Could you check a few things on this model? Use its own coordinates, in mm. A direction names the side the tool comes from. Give positions to 0.01 mm unless a question says otherwise; leave off trailing zeros. Order: outer loops, then holes, each group sorted by start corner. A loop starts at its lowest first (then second) coordinate and runs counter-clockwise, first axis right, second up. Notation, with made-up numbers: M 74.5,-16 L 93.5,-16 A19 ccw 93.5,-7 Z; hole C 11,-18 d4. An arc over 180 degrees is marked long. Answer in a Markdown table with one row per item. Add a question column.
Autodesk Inventor part; units mm, degrees
ref_plane "YZ Plane" through (0, 0, 0) normal (1, 0, 0) x (0, 1, 0)
ref_plane "XZ Plane" through (0, 0, 0) normal (0, 1, 0) x (-1, 0, 0)
ref_plane "XY Plane" through (0, 0, 0) normal (0, 0, 1) x (1, 0, 0)
sketch "Boceto1" plane through (0, 0, 0) normal (0, 0, 1) x (1, 0, 0)
  line L0 (0, 0) -> (42, 0)
  line L1 (42, 0) -> (42, 42)
  line L2 (42, 42) -> (35, 42)
  line L3 (35, 42) -> (35, 7)
  line L4 (35, 7) -> (0, 7)
  line L5 (0, 7) -> (0, 0)
  dimension "d0" = 7
  dimension "d1" = 7
  dimension "d2" = 42
  dimension "d3" = 42
extrude "Extrusión1" add sketch "Boceto1" along normal blind 41.5
sketch "Boceto2" plane through (0, 0, 41.5) normal (0, 0, 1) x (1, 0, 0)
  line L0 (35, 7) -> (0, 7)
  line L1 (35, 7) -> (35, 38)
  line L2 (35, 42) -> (35, 7)
  line L3 (35, 38) -> (4, 7)
  line L4 (4, 7) -> (35, 7)
  line L5 (42, 42) -> (35, 42)
  point P0 (0, 0)
  point P1 (4, 7)
  dimension "d6" = 4
  dimension "d7" = 4
extrude "Extrusión2" add sketch "Boceto2" against normal blind 4
sketch "Boceto3" plane through (0, 0, 0) normal (0, 0, -1) x (-1, 0, 0)
  line L0 (-4, 7) -> (-35, 38)
  line L1 (-35, 42) -> (-35, 7)
  line L2 (-35, 7) -> (0, 7)
  point P0 (0, 0)
extrude "Extrusión3" add sketch "Boceto3" against normal blind 4
sketch "Boceto4" plane through (35, 42, 0) normal (-1, 0, 0) x (0, 0, 1)
  line L0 (20.75, -11.35) -> (20.75, -22.65) construction
  line L1 (16.4, -11.35) -> (16.4, -22.65)
  line L2 (25.1, -22.65) -> (25.1, -11.35)
  arc A0 (25.1, -11.35) -> (16.4, -11.35) centre (20.75, -11.35) ccw
  arc A1 (16.4, -22.65) -> (25.1, -22.65) centre (20.75, -22.65) ccw
  line L3 (0, 0) -> (41.5, 0)
  point P0 (0, -42)
  point P1 (20.75, -17)
  point P2 (20.75, 0)
  point P3 (20.75, -27)
  point P4 (20.75, -7)
  dimension "d12" = 8.7
  dimension "d13" = 20
  dimension "d14" = 7
extrude "Extrusión4" cut sketch "Boceto4" against normal through all
sketch "Boceto5" plane through (0, 7, 41.5) normal (0, 1, 0) x (1, 0, 0)
  line L0 (22.65, 20.75) -> (11.35, 20.75) construction
  line L1 (22.65, 25.1) -> (11.35, 25.1)
  line L2 (11.35, 16.4) -> (22.65, 16.4)
  arc A0 (22.65, 16.4) -> (22.65, 25.1) centre (22.65, 20.75) ccw
  arc A1 (11.35, 25.1) -> (11.35, 16.4) centre (11.35, 20.75) ccw
  line L3 (0, 41.5) -> (0, 0)
  point P0 (17, 20.75)
  point P1 (0, 20.75)
  point P2 (27, 20.75)
  point P3 (7, 20.75)
  dimension "d17" = 20
  dimension "d18" = 7
  dimension "d19" = 8.7
extrude "Extrusión5" cut sketch "Boceto5" against normal blind 10
properties part number "escuadra pequeña"
1. Suppose I cut it at D-D on x = 8. List the corners of the cut face in (y, z) for me.
2. Thinking about a two-plate mould opening in Y: for faces 1 (the flat face through (21, 0, 16)), 2 (the flat face through (38, 25, 16.4)), 3 (the cylindrical face through (38.5, 35, 20.8)), 4 (the flat face through (27, 16, 4)), which applies, pulls with the +Y half, pulls with the -Y half, needs draft (parallel to the pull), parting line crosses it, or undercut?
3. Suppose I cut it at A-A on z = 20.75. List the corners of the cut face in (x, y) for me, plus the area to 3 significant figures.
4. Will these pins go through, and if not, where does the flat tip stop? P1, Ø5, axis at x = 26.5, z = 15.5, coming from the -Y side; P2, Ø8, axis at x = 8, y = 18, coming from the +Z side; P3, Ø8, axis at y = 35, z = 20.5, coming from the -X side.
5. Suppose I cut it at B-B on x = 36. List the corners of the cut face in (y, z) for me.
6. For faces 5 (the cylindrical face through (38.5, 15, 20.7)), 6 (the flat face through (42, 21, 16)), 7 (the flat face through (35, 25, 16)), 8 (the cylindrical face through (7, 3.5, 20.7)), which set-ups out of +Z, -Z, +X, -X, +Y, -Y let a thin tool reach every point of the face, with its end or its side?
7. Suppose I cut it at C-C on y = 26.5. List the corners of the cut face in (x, z) for me.
8. If I drill on line 1 along Z through (x, y) = (27, 18); line 2 along Z through (x, y) = (18.5, 4); line 3 along Y through (x, z) = (28, 12), over which ranges is the centre line in solid material (lowest first)? Write a range as [from, to].
Findings below:
| question | item | result |
|---|---|---|
| 1 | outline | M 0,0 L 11,0 L 11,4 L 7,4 L 7,17.98 L 0,17.98 Z; M 0,23.52 L 7,23.52 L 7,37.5 L 11,37.5 L 11,41.5 L 0,41.5 Z |
| 2 | face 1 | pulls with the -Y half |
| 2 | face 2 | undercut |
| 2 | face 3 | undercut |
| 2 | face 4 | needs draft |
| 3 | outline | M 0,0 L 7,0 L 7,7 L 0,7 Z; M 27,0 L 42,0 L 42,15 L 35,15 L 35,7 L 27,7 Z; M 35,35 L 42,35 L 42,42 L 35,42 Z |
| 3 | area | 259 mm2 |
| 4 | P1 | y = 0 |
| 4 | P2 | through |
| 4 | P3 | x = 35 |
| 5 | outline | M 0,0 L 42,0 L 42,41.5 L 0,41.5 Z; hole M 19.35,16.4 L 30.65,16.4 A4.35 ccw 30.65,25.1 L 19.35,25.1 A4.35 ccw Z |
| 6 | face 5 | +X, -X |
| 6 | face 6 | +Z, -Z, +X, +Y, -Y |
| 6 | face 7 | -X, +Y |
| 6 | face 8 | +Y, -Y |
| 7 | outline | M 23.5,0 L 42,0 L 42,16.4 L 35,16.4 L 35,4 L 23.5,4 Z; M 23.5,37.5 L 35,37.5 L 35,25.1 L 42,25.1 L 42,41.5 L 23.5,41.5 Z |
| 8 | line 1 | [0, 4], [37.5, 41.5] |
| 8 | line 2 | [0, 16.4], [25.1, 41.5] |
| 8 | line 3 | [0, 7] |
